from build123d import *

# Parameters (mm, degrees)
F0_R     = 36.1502076958
F1_DEPTH = 25
F3_DEPTH = 25


with BuildPart() as f1:
    # F0 (on Top) → F1 (new body)
    with BuildSketch(Plane.XY):
        Circle(F0_R)
    extrude(amount=F1_DEPTH)

    # F2 (on face) → F3 (cut)
    with BuildSketch(Plane.XY.offset(25)):
        with BuildLine():
            Line((-8.2388771698, 0), (0, 0))
            Line((0, 0), (0, 36.1502076958))
            ThreePointArc((0, 36.1502076958), (-7.0998109764, 35.4461591791), (-13.9230751939, 33.3614372232))
            Line((-13.9230751939, 33.3614372232), (-9.4486636828, 19.5610804365))
            Line((-9.4486636828, 19.5610804365), (-4.2720828205, 15.8297549933))
            Line((-4.2720828205, 15.8297549933), (-8.2388771698, 10.326500982))
            Line((-8.2388771698, 10.326500982), (-8.2388771698, 0))
        make_face()
        with BuildLine():
            Line((0, 36.1502076958), (0, 0))
            Line((0, 0), (7.1280188859, 0))
            Line((7.1280188859, 0), (7.1280188859, 10.326500982))
            Line((7.1280188859, 10.326500982), (3.5276915878, 15.274326317))
            Line((3.5276915878, 15.274326317), (8.1382541345, 19.5610804365))
            Line((8.1382541345, 19.5610804365), (11.5974145733, 34.2394143008))
            ThreePointArc((11.5974145733, 34.2394143008), (5.8768859991, 35.6693107223), (0, 36.1502076958))
        make_face()
    extrude(amount=-F3_DEPTH, mode=Mode.SUBTRACT)


solid = f1.part
CAD build for the part. Positions are in the model's coordinates, mm. A direction names the side the tool comes from. Coordinates: 2 decimals unless noted, no trailing zeros. Write each loop counter-clockwise with the first axis right and the second up, starting at its lowest first coordinate (ties: lowest second). Pieces come first, ordered by that corner, then holes. Notation, with made-up numbers: (70, 83) - (98, 83) arc R35 ccw to (98, 115) - close; hole circle Ø9 at (21, -8). An arc over 180 degrees is marked (long way). Use a Markdown table: item, result. Add a question column.
Item 1: Flat gauge pins, fed straight in: pin 1 (2 mm diameter, centred on y = -16, z = 7, fed in from -X); pin 2 (8.5 mm diameter, centred on y = 7.5, z = 15, fed in from -X); pin 3 (8.5 mm diameter, centred on y = 7, z = 14, fed in from +X). Where does each tip first touch, or does it go through?
Item 2: Drill centre lines: L1, parallel to X at y = 1, z = 1.25; L2, parallel to Y at x = 0.5, z = 8; L3, parallel to X at y = 22, z = 18. Where is each one in solid material? Low to high. Write a range as from..to.
Item 3: Band-saw the part on B-B, the plane y = 3.5. Give the cut face in (x, z), and give its area (3 significant figures).
Item 4: Band-saw the part on A-A, the plane z = 22.75. Give the cut face in (x, y).
Item 5: Band-saw the part on C-C, the plane x = 0. Give the cut face in (y, z), and give its area (3 significant figures).
Item 6: 3-axis set-ups, long thin cutter, end or side, ignore diameter. For faces 5 (the face through (-8.239, 5, 13)), 6 (the face through (-0.5, -0.5, 25)), 7 (the face through (5.801, 17.388, 12.675)): which of +Z, -Z, +X, -X, +Y, -Y reach the whole face in a straight line?
Item 7: Mould opens along Y. For faces 1 (the face through (-11.717, 26.558, 12.675)), 2 (the face through (5.35, 12.77, 12.68)), 3 (the face through (7.128, 5, 13)), 4 (the face through (-0.5, -0.5, 0)) say: pulls with the +Y half, pulls with the -Y half, needs draft (parallel to the pull), parting line crosses it, or undercut.
Item 8: Band-saw the part on D-D, the plane y = -23. Give the cut face in (x, z), and give its area (3 significant figures).
Numbers:
| question | item | result |
|---|---|---|
| 1 | pin 1 | x = -32.89 |
| 1 | pin 2 | x = -36 |
| 1 | pin 3 | x = 36.05 |
| 2 | L1 | -36.14..-8.24, 7.13..36.14 |
| 2 | L2 | -36.15..0 |
| 2 | L3 | -28.69..-10.24, 8.71..28.69 |
| 3 | outline | (-35.98, 0) - (-8.24, 0) - (-8.24, 25) - (-35.98, 25) - close; (7.13, 0) - (35.98, 0) - (35.98, 25) - (7.13, 25) - close |
| 3 | area | 1,410 mm2 |
| 4 | outline | (-13.92, 33.36) arc R36.15 ccw (long way) to (11.6, 34.24) - (8.14, 19.56) - (3.53, 15.27) - (7.13, 10.33) - (7.13, 0) - (-8.24, 0) - (-8.24, 10.33) - (-4.27, 15.83) - (-9.45, 19.56) - close |
| 5 | outline | (-36.15, 0) - (0, 0) - (0, 25) - (-36.15, 25) - close |
| 5 | area | 904 mm2 |
| 6 | face 5 | +Z, -Z |
| 6 | face 6 | +Z, +X, -X, +Y, -Y |
| 6 | face 7 | +Z, -Z, +Y |
| 7 | face 1 | pulls with the +Y half |
| 7 | face 2 | undercut |
| 7 | face 3 | undercut |
| 7 | face 4 | needs draft |
| 8 | outline | (-27.89, 0) - (27.89, 0) - (27.89, 25) - (-27.89, 25) - close |
| 8 | area | 1,390 mm2 |
